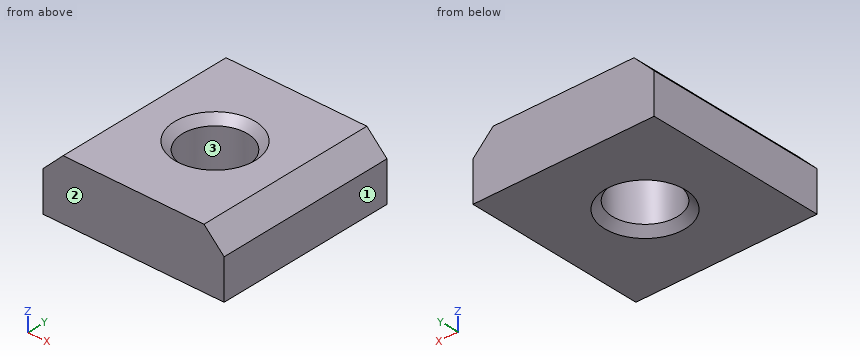
Autodesk Inventor part; units mm, degrees
ref_plane "YZ Plane" through (0, 0, 0) normal (1, 0, 0) x (0, 1, 0)
ref_plane "XZ Plane" through (0, 0, 0) normal (0, 1, 0) x (-1, 0, 0)
ref_plane "XY Plane" through (0, 0, 0) normal (0, 0, 1) x (1, 0, 0)
sketch "Sketch_1" plane through (0, 0, 0) normal (0, 0, 1) x (1, 0, 0)
  line L0 (-4.5, 4.5) -> (-4.5, -4.5)
  line L1 (-4.5, -4.5) -> (4.5, -4.5)
  line L2 (4.5, -4.5) -> (4.5, 4.5)
  line L3 (4.5, 4.5) -> (-4.5, 4.5)
extrude "Extrusion1" add sketch "Sketch_1" along normal mid plane 3
sketch "Sketch_2" plane through (0, 0, 0) normal (1, 0, 0) x (0, 1, 0)
  line L0 (0, -1.5) -> (0, 1.5)
  line L1 (0, 1.5) -> (2, 1.5)
  line L2 (2, 1.5) -> (1.621, 1.121)
  line L3 (1.621, 1.121) -> (1.621, -1.121)
  line L4 (1.621, -1.121) -> (2, -1.5)
  line L5 (2, -1.5) -> (0, -1.5)
  line L6 (0, -1.5) -> (0, 1.5)
revolve "Revolution1" cut sketch "Sketch_2" angle 360 about axis through (0, 0, -1.5) along (0, 0, -1)
thread "Thread1"
sketch "Sketch_3" plane through (0, 0, 0) normal (0, 1, 0) x (-1, 0, 0)
  line L0 (4.5, 0.5) -> (4.5, 2.5)
  line L1 (4.5, 2.5) -> (-4.5, 2.5)
  line L2 (-4.5, 2.5) -> (-4.5, 0.5)
  line L3 (-4.5, 0.5) -> (-3.5, 1.5)
  line L4 (-3.5, 1.5) -> (3.5, 1.5)
  line L5 (3.5, 1.5) -> (4.5, 0.5)
extrude "Extrusion2" cut sketch "Sketch_3" along normal mid plane 18
properties part number "14159_m"
Design review of the part built by this model. Coordinates are the model's own, in mm. Face numbers are marked on the shaded views. Coordinates: 2 decimals unless noted, no trailing zeros. Loops run counter-clockwise (first coordinate to the right, second up) from the corner with the lowest first, then second, coordinate; pieces in that order, holes last. Notation, with made-up numbers: (-23, 49.25) - (20, 49.25) arc R21 cw to (20, 72.25) - close; hole circle Ø9 at (11.5, 38). An arc over 180 degrees is marked (long way). Use CSV: the item, a comma, the result in double quotes. Start each with the question number.
1) The part is to be moulded in two halves that separate along Y. For the marked faces 1, 2 and 3, say which applies: +Y half, -Y half, draft (parallel to the pull), parting line (faces both ways), or undercut.
2) Consider section D-D on y = 2.25. Write out the cut boundary in (x, z).
3) Consider section A-A on y = 0. Write out the cut boundary in (x, z).
4) For pin 1 Ø3 at (x, y) = (0, 0) entering from -Z, flat-tipped, find the tip position at first contact; note if it passes through.
5) Wall thickness on L1, parallel to X at y = 0, z = 0.35; L2, parallel to X at y = 0.75, z = -0.9: over which ranges is each line inside the solid? List them lowest first. Write a range as from..to.
6) Consider section C-C on z = 0.1. Write out the cut boundary in (x, y).
7) Consider section B-B on x = 0. Write out the cut boundary in (y, z).
Geometry says:
1,face 1,"draft"
1,face 2,"-Y half"
1,face 3,"undercut"
2,outline,"(-4.5, -1.5) - (4.5, -1.5) - (4.5, 0.5) - (3.5, 1.5) - (-3.5, 1.5) - (-4.5, 0.5) - close"
3,outline,"(-4.5, -1.5) - (-2, -1.5) - (-1.62, -1.12) - (-1.62, 1.12) - (-2, 1.5) - (-3.5, 1.5) - (-4.5, 0.5) - close; (1.62, -1.12) - (2, -1.5) - (4.5, -1.5) - (4.5, 0.5) - (3.5, 1.5) - (2, 1.5) - (1.62, 1.12) - close"
4,pin 1,"through"
5,L1,"-4.5..-1.62, 1.62..4.5"
5,L2,"-4.5..-1.44, 1.44..4.5"
6,outline,"(-4.5, -4.5) - (4.5, -4.5) - (4.5, 4.5) - (-4.5, 4.5) - close; hole circle Ø3.24 at (0, 0)"
7,outline,"(-4.5, -1.5) - (-2, -1.5) - (-1.62, -1.12) - (-1.62, 1.12) - (-2, 1.5) - (-4.5, 1.5) - close; (1.62, -1.12) - (2, -1.5) - (4.5, -1.5) - (4.5, 1.5) - (2, 1.5) - (1.62, 1.12) - close"
